Could you check a few things on this model? Use its own coordinates, in mm. Face numbers are marked on the shaded views. A direction names the side the tool comes from. Round coordinates to 2 decimals unless told otherwise and drop trailing zeros. Order: outer loops, then holes, each group sorted by start corner. A loop starts at its lowest first (then second) coordinate and runs counter-clockwise, first axis right, second up. Notation, with made-up numbers: M 80,-26 L 124,-26 A26 ccw 124,-3 Z; hole C 16.5,30 d10. An arc over 180 degrees is marked long. Write each question's results on one line, items separated by ' | '. Start each with the question number.
1. Suppose I cut it at A-A on x = 0. Write out the boundary of the cut face in (y, z), and give its area (3 significant figures).
2. For the marked faces 1 and 2, which set-ups out of +Z, -Z, +X, -X, +Y, -Y let a thin tool reach every point of the face, with its end or its side?
3. Suppose I cut it at C-C on z = -9.5. Write out the boundary of the cut face in (x, y), and give its area (3 significant figures).
4. I'm going to push flat-ended pins straight in: pin 1 (8 mm diameter, centred on y = -4, z = -35, fed in from -X); pin 2 (12 mm diameter, centred on y = 3.5, z = -30.5, fed in from +X); pin 3 (12 mm diameter, centred on x = -2.5, z = -9.5, fed in from -Y). Where does each tip first touch, or does it pass through?
5. Please list where these lines run through material, in increasing order: L1, parallel to Y at x = -5.5, z = -26.5; L2, parallel to Y at x = 2.5, z = -4.5; L3, parallel to X at y = -10.5, z = -54.
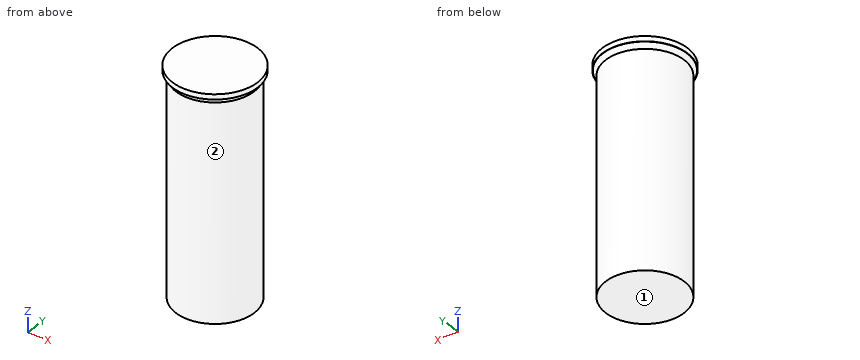
from build123d import *

# Parameters (mm, degrees)
F0_R     = 12.5
F1_DEPTH = 1.5
F3_DEPTH = 1.5
F4_DEPTH = 63


# Not quite as in the source:
# - a fillet or chamfer that OpenCascade refuses, or shapes differently, is made with other operations: its cross-section is extruded or revolved along the edge and cut away or added


with BuildPart() as f1:
    # F0 (on Top) → F1 (new body)
    with BuildSketch(Plane.XY):
        Circle(F0_R)
    extrude(amount=-F1_DEPTH)

    # F2: chamfer of 1 x 1.7320508076 on 1 edges, made by hand

    # F2_s1 → F2_t2 (revolve, cut)
    with BuildSketch(Plane.XZ):
        Polygon((12.5, 0.2320508076), (11.5, -1.5), (12.5, -1.5), align=None)
    revolve(axis=Axis((0, 0, -1.5), (0, 0, 1)), mode=Mode.SUBTRACT)

    # F0 (on Top) → F3 (join)
    with BuildSketch(Plane.XY):
        Circle(F0_R)
    extrude(amount=F3_DEPTH)

    # F4 (add): a face of the model
    f4_faces = [f1.faces().sort_by_distance(p)[0] for p in [
        (0, 0, -1.5),
    ]]
    extrude(f4_faces, amount=F4_DEPTH)


solid = f1.part
Filled sheet:
1) outline: M -12.5,0 L -12.37,0 L -11.5,-1.5 L -11.5,-64.5 L 11.5,-64.5 L 11.5,-1.5 L 12.37,0 L 12.5,0 L 12.5,1.5 L -12.5,1.5 Z | area: 1,520 mm^2
2) face 1: -Z, +X, -X, +Y, -Y | face 2: -Z
3) outline: C 0,0 d23 | area: 415 mm^2
4) pin 1: stops at x = -11.5 | pin 2: stops at x = 11.5 | pin 3: stops at y = -11.5
5) L1: y = -10.1 to 10.1 | L2: y = -11.22 to 11.22 | L3: x = -4.69 to 4.69
